Autodesk Inventor part; units mm, degrees
ref_plane "YZ Plane" through (0, 0, 0) normal (1, 0, 0) x (0, 1, 0)
ref_plane "XZ Plane" through (0, 0, 0) normal (0, 1, 0) x (-1, 0, 0)
ref_plane "XY Plane" through (0, 0, 0) normal (0, 0, 1) x (1, 0, 0)
sketch "スケッチ1" plane through (0, 0, 0) normal (1, 0, 0) x (0, 1, 0)
  line L0 (10, 0) -> (10, -12)
  line L1 (22, -12) -> (22, -7)
  line L2 (22, -7) -> (20, -7)
  line L3 (20, -7) -> (20, 0)
  line L4 (20, 0) -> (10, 0)
  line L5 (0, -14.4) -> (0, 2.4)
  line L6 (22, -12) -> (10, -12)
  point P0 (0, 0)
  dimension "d0" = 20
  dimension "d1" = 2
  dimension "d2" = 7
  dimension "d3" = 5
  dimension "d4" = 10
revolve "回転1" add sketch "スケッチ1" angle 360 about axis through (0, 0, -10) along (0, 0, 1)
sketch "スケッチ2" plane through (0, 0, 0) normal (0, 0, 1) x (1, 0, 0)
  circle A0 centre (0, 0) radius 20
  circle A1 centre (0, 0) radius 15
  point P0 (0, 15)
  point P1 (-12.9904, 7.5)
  point P2 (-12.9904, -7.5)
  point P3 (0, -15)
  point P4 (12.9904, -7.5)
  point P5 (12.9904, 7.5)
  dimension "d8" = 5
  dimension "d11" = 360
hole "穴1" at (0, 15, 0) at (-12.9904, 7.5, 0) at (-12.9904, -7.5, 0) at (0, -15, 0) at (12.9904, -7.5, 0) at (12.9904, 7.5, 0) direction (0, 0, -1) diameter 3.2 end through all
chamfer "面取り1" distance 1 angle 45 1 edges at (0, -20, 0)
properties part number "base1" material "ABS プラスチック"
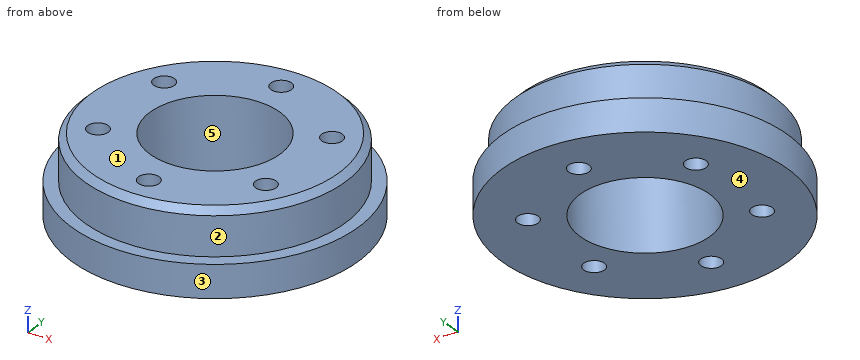
Design review of the part built by this model. Coordinates are the model's own, in mm. Face numbers are marked on the shaded views. A direction names the side the tool comes from. Round coordinates to 2 decimals unless told otherwise and drop trailing zeros. Write each loop counter-clockwise with the first axis right and the second up, starting at its lowest first coordinate (ties: lowest second). Pieces come first, ordered by that corner, then holes. Notation, with made-up numbers: (13, 10) - (45, 10) arc R16 cw to (45, 23) - close; hole circle Ø11 at (-24.5, 45.25). An arc over 180 degrees is marked (long way). Use a Markdown table: item, result. Add a question column.
1. Clearance check with flat-ended pins moving along their axes: pin 1 (1.5 mm diameter, centred on x = -4, z = -6.5, fed in from -Y); pin 2 (2 mm diameter, centred on x = 7, z = -3, fed in from -Y); pin 3 (5 mm diameter, centred on y = 4.5, z = -2.5, fed in from -X). State where each tip first meets the part, or that it passes through.
2. We need section C-C (y = -7.5). Count the separate pieces of the cut face and the enclosed holes in it, then the cut area to 3 significant figures.
3. Wall thickness on probe 1 along Y at (x, z) = (0, -8.25); probe 2 along Y at (x, z) = (12.5, -3); probe 3 along Y at (x, z) = (-14, -2.25): over which ranges is each line inside the solid? List them lowest first.
4. We need section A-A (y = 0). State the section outline as (x, z) points.
5. We need section B-B (z = -5.5). State the section outline as (x, y) points, then the cut area to 3 significant figures.
6. Mouldability with a two-part tool opening along X and no side actions: class the marked faces 3, 4 and 5 as +X half, -X half, draft (parallel to the pull), parting line (faces both ways), or undercut.
7. For the marked faces 1 and 2, list the 3-axis set-ups (+Z, -Z, +X, -X, +Y, -Y) from which the entire face can be reached by the end or side of a thin tool; tool diameter is ignored.
Output:
| question | item | result |
|---|---|---|
| 1 | pin 1 | stops at y = -21.73 |
| 1 | pin 2 | stops at y = -19.08 |
| 1 | pin 3 | stops at x = -19.9 |
| 2 | separate pieces | 4 |
| 2 | enclosed holes | 0 |
| 2 | area | 230 mm2 |
| 3 | probe 1 | y = -22 to -16.6, -13.4 to -10, 10 to 13.4, 16.6 to 22 |
| 3 | probe 2 | y = -15.61 to -9.02, -5.98 to 5.98, 9.02 to 15.61 |
| 3 | probe 3 | y = -14.28 to -8.74, -6.26 to 6.26, 8.74 to 14.28 |
| 4 | outline | (-22, -12) - (-10, -12) - (-10, 0) - (-19, 0) - (-20, -1) - (-20, -7) - (-22, -7) - close; (10, -12) - (22, -12) - (22, -7) - (20, -7) - (20, -1) - (19, 0) - (10, 0) - close |
| 5 | outline | circle Ø40 at (0, 0); hole circle Ø3.2 at (-12.99, -7.5); hole circle Ø3.2 at (-12.99, 7.5); hole circle Ø20 at (0, 0); hole circle Ø3.2 at (0, -15); hole circle Ø3.2 at (0, 15); hole circle Ø3.2 at (12.99, -7.5); hole circle Ø3.2 at (12.99, 7.5) |
| 5 | area | 894 mm2 |
| 6 | face 3 | parting line |
| 6 | face 4 | draft |
| 6 | face 5 | undercut |
| 7 | face 1 | +Z, +X, -X, +Y, -Y |
| 7 | face 2 | +Z |
